Could you check a few things on this model? Use its own coordinates, in mm. Face numbers are marked on the shaded views. A direction names the side the tool comes from. Round coordinates to 2 decimals unless told otherwise and drop trailing zeros. Loops run counter-clockwise (first coordinate to the right, second up) from the corner with the lowest first, then second, coordinate; pieces in that order, holes last. Notation, with made-up numbers: (62, 7.25) -> (97, 7.25) arc R34 cw to (97, 41.25) -> close; hole circle Ø8 at (55, 46.5). An arc over 180 degrees is marked (long way). Write each question's results on one line, items separated by ' | '.
from build123d import *

# Parameters (mm, degrees)
F1_DEPTH = 5
F2_W     = 5
F2_H     = 94
F3_DEPTH = 12
F5_DEPTH = 5
F8_DEPTH = 5


with BuildPart() as f1:
    # F0 (on Top) → F1 (new body)
    with BuildSketch(Plane.XY):
        Polygon((-8.5, -47), (8.5, -47), (8.5, 47), (3.75, 47), (1.25, 47), (-8.5, 47), align=None)
    extrude(amount=F1_DEPTH)

    # F2 (on face) → F3 (join)
    with BuildSketch(Plane.XY.offset(5)):
        with Locations((-6, 0)):
            Rectangle(F2_W, F2_H)
    extrude(amount=F3_DEPTH)


with BuildPart() as f5:
    # F4 (on face) → F5 (new body)
    with BuildSketch(Plane.YZ.offset(-3.5)):
        Polygon((50.75, 13.5), (47, 12.25), (47, 9.75), (50.75, 8.5), align=None)
    extrude(amount=-F5_DEPTH)


with BuildPart() as f1_1:
    add(f1.part)

    # F6: union F5
    add(f5.part)

    # F7 (on face) → F8 (cut)
    with BuildSketch(Plane.YZ.offset(-3.5)):
        Polygon((-47, 12.25), (-47, 9.75), (-43.25, 8.5), (-43.25, 13.5), align=None)
    extrude(amount=-F8_DEPTH, mode=Mode.SUBTRACT)


solid = f1_1.part
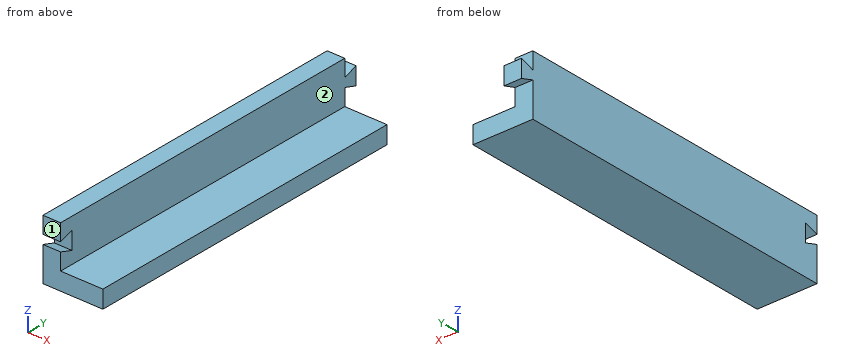
1) I want a section at B-B, the plane x = 5.75. Write out the boundary of the cut face in (y, z).
Model answer:
outline: (-47, 0) -> (47, 0) -> (47, 5) -> (-47, 5) -> close
2) I want a section at C-C, the plane z = 3.5. Write out the boundary of the cut face in (x, y).
Model answer:
outline: (-8.5, -47) -> (8.5, -47) -> (8.5, 47) -> (-8.5, 47) -> close
3) I need wall thicknesses on line 1 (X direction, y = -36.5, z = 7.5); line 2 (Z direction, x = -1.5, y = 39); line 3 (Y direction, x = -5.75, z = 5.25). Which ranges of each line are inside material? Lowest first, please.
Model answer:
line 1: x = -8.5 to -3.5 | line 2: z = 0 to 5 | line 3: y = -47 to 47
4) I want a section at A-A, the plane y = 0.5. Write out the boundary of the cut face in (x, z).
Model answer:
outline: (-8.5, 0) -> (8.5, 0) -> (8.5, 5) -> (-3.5, 5) -> (-3.5, 17) -> (-8.5, 17) -> close
5) I'm going to push flat-ended pins straight in: pin 1 (2 mm diameter, centred on x = 0, y = -10, fed in from +Z); pin 2 (8 mm diameter, centred on x = -6, z = 2, fed in from +Y); pin 3 (3.5 mm diameter, centred on y = 22.5, z = 8.5, fed in from +X). Where does each tip first touch, or does it pass through?
Model answer:
pin 1: stops at z = 5 | pin 2: stops at y = 47 | pin 3: stops at x = -3.5
6) For the marked faces 1 and 2, which set-ups out of +Z, -Z, +X, -X, +Y, -Y let a thin tool reach every point of the face, with its end or its side?
Model answer:
face 1: +Z, -Z, +X, -X, -Y | face 2: +Z, +X, +Y, -Y
